Check sheet for the modelled part. Datum: model origin and axes. Units: mm. Face numbers are marked on the shaded views. A direction names the side the tool comes from. Round coordinates to 2 decimals unless told otherwise and drop trailing zeros. Order: outer loops, then holes, each group sorted by start corner. A loop starts at its lowest first (then second) coordinate and runs counter-clockwise, first axis right, second up.
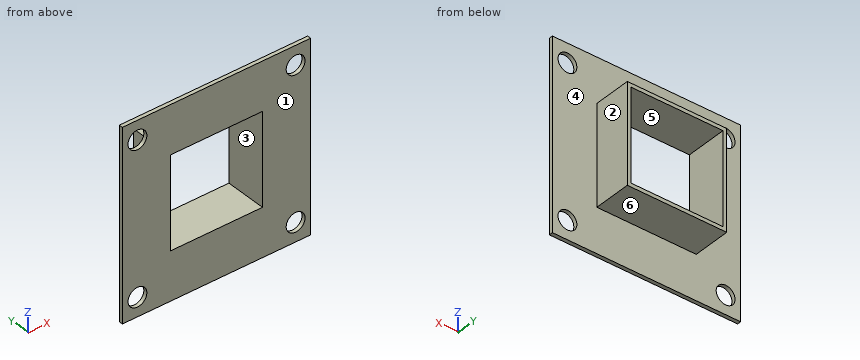
from build123d import *

# Parameters (mm, degrees)
SKETCH1_W           = 67.056
SKETCH1_H           = 67.056
SKETCH1_W_2         = 61.976
SKETCH1_H_2         = 61.976
BOSS_EXTRUDE1_DEPTH = 25.4
SKETCH3_W           = 127
SKETCH3_H           = 127
BOSS_EXTRUDE2_DEPTH = 2.54
SKETCH4_R           = 6.35
CUT_EXTRUDE1_DEPTH  = 94.3255592
SKETCH6_W           = 61.976
SKETCH6_H           = 61.976
CUT_EXTRUDE2_DEPTH  = 94.3255592


with BuildPart() as part:
    # Sketch1 → Boss-Extrude1 (new body)
    with BuildSketch(Plane(origin=(0, 0, 0), x_dir=(1, 0, 0), z_dir=(0, 1, 0))):
        Rectangle(SKETCH1_W, SKETCH1_H)
        Rectangle(SKETCH1_W_2, SKETCH1_H_2, mode=Mode.SUBTRACT)
    extrude(amount=BOSS_EXTRUDE1_DEPTH)

    # Sketch3 → Boss-Extrude2 (add)
    with BuildSketch(Plane.XZ):
        Rectangle(SKETCH3_W, SKETCH3_H)
    extrude(amount=BOSS_EXTRUDE2_DEPTH)

    # Sketch4 → Cut-Extrude1 (cut, through all)
    with BuildSketch(Plane(origin=(0, 0, 0), x_dir=(1, 0, 0), z_dir=(0, 1, 0))):
        with Locations(Location((-53.34, 50.8, 0), (0, 0, 270))):
            Circle(SKETCH4_R)
        with Locations(Location((53.34, 50.8, 0), (0, 0, 270))):
            Circle(SKETCH4_R)
        with Locations(Location((53.34, -50.8, 0), (0, 0, 270))):
            Circle(SKETCH4_R)
        with Locations(Location((-53.34, -50.8, 0), (0, 0, 270))):
            Circle(SKETCH4_R)
    extrude(amount=-CUT_EXTRUDE1_DEPTH, mode=Mode.SUBTRACT)

    # Sketch6 → Cut-Extrude2 (cut, through all)
    with BuildSketch(Plane(origin=(0, 0, 0), x_dir=(1, 0, 0), z_dir=(0, 1, 0))):
        Rectangle(SKETCH6_W, SKETCH6_H)
    extrude(amount=-CUT_EXTRUDE2_DEPTH, mode=Mode.SUBTRACT)


solid = part.part
1) Sectioned sample at A-A on z = 17.5. Record the cut outline in (x, y).
2) Scan lines: line 1 (X direction, y = -1.85, z = -50.8); line 2 (Z direction, x = -19.5, y = 11). Record each from-to range of solid material in increasing order.
3) Draft check along Z on the marked faces 4, 5 and 6. Enter one of: pulls with the +Z half, pulls with the -Z half, needs draft (parallel to the pull), parting line crosses it, or undercut.
4) Sectioned sample at D-D on z = 51.5. Record the cut outline in (x, y).
5) Set-up check for the marked faces 1, 2 and 3: record each of +Z, -Z, +X, -X, +Y, -Y from which the full face is reachable in a straight line by a thin tool's end or side.
6) Sectioned sample at B-B on x = 5. Record the cut outline in (y, z).
7) Gauge pin test, flat ends, axial feed: pin 1 (8 mm diameter, centred on y = 22, z = 39, fed in from +X); pin 2 (12 mm diameter, centred on y = 18.5, z = -26, fed in from +X); pin 3 (7.5 mm diameter, centred on x = -4.5, y = 7.5, fed in from -Z); pin 4 (1.5 mm diameter, centred on x = 34, y = 17.5, fed in from +Z). Record the tip position at first contact, or that the pin passes through.
8) Sectioned sample at C-C on y = 11.25. Record the cut outline in (x, z), and give its area (3 significant figures).
Values found:
1. outline: (-63.5, -2.54) - (-30.99, -2.54) - (-30.99, 25.4) - (-33.53, 25.4) - (-33.53, 0) - (-63.5, 0) - close; (30.99, -2.54) - (63.5, -2.54) - (63.5, 0) - (33.53, 0) - (33.53, 25.4) - (30.99, 25.4) - close
2. line 1: x = -63.5 to -59.69, -46.99 to 46.99, 59.69 to 63.5
2. line 2: z = -33.53 to -30.99, 30.99 to 33.53
3. face 4: needs draft
3. face 5: undercut
3. face 6: pulls with the -Z half
4. outline: (-63.5, -2.54) - (-59.65, -2.54) - (-59.65, 0) - (-63.5, 0) - close; (-47.03, -2.54) - (47.03, -2.54) - (47.03, 0) - (-47.03, 0) - close; (59.65, -2.54) - (63.5, -2.54) - (63.5, 0) - (59.65, 0) - close
5. face 1: +Z, -Z, +X, -X, -Y
5. face 2: +Z, -Z, +X, +Y
5. face 3: +Y, -Y
6. outline: (-2.54, -63.5) - (0, -63.5) - (0, -33.53) - (25.4, -33.53) - (25.4, -30.99) - (-2.54, -30.99) - close; (-2.54, 30.99) - (25.4, 30.99) - (25.4, 33.53) - (0, 33.53) - (0, 63.5) - (-2.54, 63.5) - close
7. pin 1: passes through
7. pin 2: stops at x = 33.53
7. pin 3: stops at z = -33.53
7. pin 4: stops at z = 33.53
8. outline: (-33.53, -33.53) - (33.53, -33.53) - (33.53, 33.53) - (-33.53, 33.53) - close; hole (-30.99, -30.99) - (30.99, -30.99) - (30.99, 30.99) - (-30.99, 30.99) - close
8. area: 655 mm2
